The model under review builds one solid part; all positions refer to its coordinate system, in mm. Face numbers are marked on the shaded views. A direction names the side the tool comes from. Coordinates: 2 decimals unless noted, no trailing zeros. Write each loop counter-clockwise with the first axis right and the second up, starting at its lowest first coordinate (ties: lowest second). Pieces come first, ordered by that corner, then holes.
1) Machinability: for the marked faces 1, 2, 3, 4 and 5, which of the approach directions +Z, -Z, +X, -X, +Y, -Y give a long, thin tool a straight path to every point of the face, cutting with its end or side? Answer none if there is none.
2) Mouldability with a two-part tool opening along Z and no side actions: class the marked faces 6, 7 and 8 as released by +Z, released by -Z, zero draft, split by the parting line, or undercut.
3) Add section D-D, the plane z = 58.5. State the section outline as (x, y) points.
4) For P1, Ø12, axis at x = 14.5, z = -4.5, coming from the +Y side; P2, Ø12, axis at y = 8, z = 9.5, coming from the -X side; P3, Ø5, axis at x = 8.5, z = 10, coming from the -Y side, all flat-tipped, find the tip position at first contact; note any pin that passes through.
5) Add section C-C, the plane z = -33. State the section outline as (x, y) points.
6) For line 1 (Z direction, x = -1.5, y = 9.5); line 2 (Y direction, x = 10.5, z = 1); line 3 (X direction, y = -0.25, z = -40.5), list the stretches that pass through material, from the lowest coordinate up.
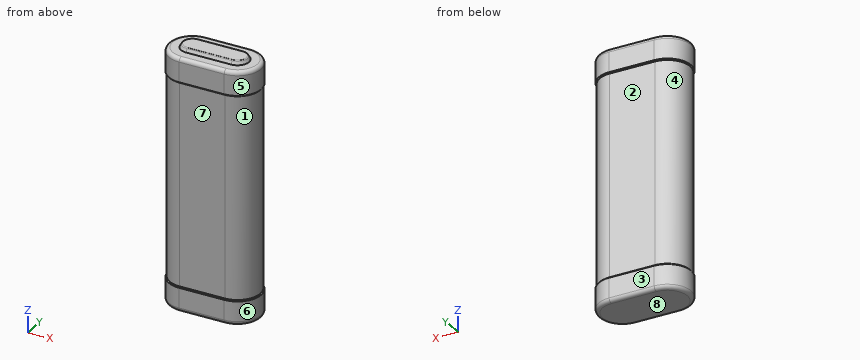
Autodesk Inventor part; units mm, degrees
ref_plane "YZ Plane" through (0, 0, 0) normal (1, 0, 0) x (0, 1, 0)
ref_plane "XZ Plane" through (0, 0, 0) normal (0, 1, 0) x (-1, 0, 0)
ref_plane "XY Plane" through (0, 0, 0) normal (0, 0, 1) x (1, 0, 0)
sketch "Sketch1" plane through (0, 0, 0) normal (0, 0, 1) x (1, 0, 0)
  arc A0 (-11.811, 11.811) -> (-11.811, -11.811) centre (-11.811, 0) ccw
  line L0 (-11.811, 11.811) -> (11.811, 11.811)
  arc A1 (11.811, -11.811) -> (11.811, 11.811) centre (11.811, 0) ccw
  line L1 (11.811, -11.811) -> (-11.811, -11.811)
  point P0 (0, 0)
  point P1 (0, 0)
extrude "Extrusion1" add sketch "Sketch1" along normal mid plane 105.41
sketch "Sketch2" plane through (0, 0, 52.705) normal (0, 0, 1) x (1, 0, 0)
  arc A0 (11.811, -12.319) -> (11.811, 12.319) centre (11.811, 0) ccw
  line L0 (11.811, -12.319) -> (-11.811, -12.319)
  arc A1 (-11.811, 12.319) -> (-11.811, -12.319) centre (-11.811, 0) ccw
  line L1 (-11.811, 12.319) -> (11.811, 12.319)
  point P0 (0, 0)
  point P1 (0, 0)
extrude "Extrusion2" add sketch "Sketch2" along normal blind 12.954
fillet "Fillet1" radius 2.032 4 edges at (-24.13, 0, 65.659) (0, 12.319, 65.659) (24.13, 0, 65.659) (0, -12.319, 65.659)
chamfer "Chamfer1" distance 0.508 angle 45 4 edges at (0, 12.319, 52.705) (24.13, 0, 52.705) (0, -12.319, 52.705) (-24.13, 0, 52.705)
mirror "Mirror1" about plane through (0, 0, 0) normal (0, 0, 1) of "Extrusion2", "Fillet1", "Chamfer1"
sketch "Sketch3" plane through (0, 0, 65.659) normal (0, 0, 1) x (1, 0, 0)
  line L0 (11.811, 5.969) -> (-11.811, 5.969)
  arc A0 (11.811, -5.969) -> (11.811, 5.969) centre (11.811, 0) ccw
  line L1 (-11.811, -5.969) -> (11.811, -5.969)
  arc A1 (-11.811, 5.969) -> (-11.811, -5.969) centre (-11.811, 0) ccw
  point P0 (0, 0)
  point P1 (11.811, 0)
  point P2 (-11.811, 0)
  point P3 (0, 0)
extrude "Extrusion3" add sketch "Sketch3" along normal blind 1.905 draft -30
fillet "Fillet2" radius 0.635 4 edges at (0, 4.8691, 67.564) (16.6801, 0, 67.564) (0, -4.8691, 67.564) (-16.6801, 0, 67.564)
properties part number "276-1491"
Geometry results:
1. face 1: +X
1. face 2: +X, -X, +Y
1. face 3: +Z, -Z, +X, -X, +Y
1. face 4: -X
1. face 5: +Z, -Z, +X
2. face 6: zero draft
2. face 7: undercut
2. face 8: released by -Z
3. outline: (-11.81, -12.32) - (11.81, -12.32) arc R12.32 ccw to (11.81, 12.32) - (-11.81, 12.32) arc R12.32 ccw to start
4. P1: stops at y = 11.81
4. P2: stops at x = -23.45
4. P3: stops at y = -11.81
5. outline: (-11.81, -11.81) - (11.81, -11.81) arc R11.81 ccw to (11.81, 11.81) - (-11.81, 11.81) arc R11.81 ccw to start
6. line 1: z = -65.66 to 65.66
6. line 2: y = -11.81 to 11.81
6. line 3: x = -23.62 to 23.62
